The listing builds one solid part. Answer for the finished solid, in the listing's coordinates (mm). A direction names the side the tool comes from. Give positions to 0.01 mm unless a question says otherwise; leave off trailing zeros. Order: outer loops, then holes, each group sorted by start corner. A loop starts at its lowest first (then second) coordinate and runs counter-clockwise, first axis right, second up. Notation, with made-up numbers: (2.25, 43) - (17.25, 43) arc R23 cw to (17.25, 74) - close; hole circle Ø3 at (75, 28). An arc over 180 degrees is marked (long way). Use a Markdown table: item, result. Add a question column.
1) The mould has two halves that part along X. Classify faces 1 (the face through (95.25, 7, 48)), 2 (the face through (8, 13, 74.885)), 3 (the face through (65.55, 4.7, 34.19)), 4 (the face through (0.724, 4.829, 94.486)): released by +X, released by -X, zero draft, split by the parting line, or undercut.
2) Find section A-A, the plane y = 12.75. Determine the outline of the cut face in (x, z) (3 decimals).
3) Flat-ended cylindrical pins translate along their axes: pin 1 (4 mm diameter, centred on x = 89.5, y = 15, fed in from -Z); pin 2 (11 mm diameter, centred on x = 9.525, z = 85.725, fed in from +Y) (3 decimals); pin 3 (3.5 mm diameter, centred on x = 11, z = 45.5, fed in from -Y). Find the tip coordinate at first contact, or state that the pin passes through.
4) Find section B-B, the plane x = 84.5. State how many separate pieces and enclosed holes the cut face has, plus the area to 3 significant figures.
5) Straight lines are drawn through the part: line 1 (Z direction, x = 47.5, y = 16.75) (3 decimals); line 2 (X direction, y = 1.5, z = 43) (3 decimals); line 3 (X direction, y = 9, z = 83). For each, find the intervals that lie inside material, in ascending order.
6) For faces 5 (the face through (46, 6.35, 13)), 6 (the face through (87, 13, 74.885)), 7 (the face through (8, 13, 20.365)), determine the directions among +Z, -Z, +X, -X, +Y, -Y from which every point of the face is accessible in a straight line to the end or side of a thin tool.
from build123d import *

# Parameters (mm, degrees)
SKETCH1_W           = 95.25
SKETCH1_H           = 95.25
SKETCH1_R           = 4.7625
BOSS_EXTRUDE1_DEPTH = 9.525
FILLET1_R           = 2.54
SKETCH3_W           = 54.519743878
SKETCH3_H           = 15.875
SKETCH3_W_2         = 15.875
SKETCH3_H_2         = 54.519743878
BOSS_EXTRUDE3_DEPTH = 7.9375
SKETCH4_R           = 3.3734375
CUT_EXTRUDE1_DEPTH  = 18.4625
SKETCH5_R           = 3.3734375
SKETCH5_W           = 0.508
SKETCH5_H           = 6.745760546
SKETCH5_W_2         = 6.745760546
SKETCH5_H_2         = 0.508
CUT_EXTRUDE2_DEPTH  = 6.35


with BuildPart() as part:
    # Sketch1 → Boss-Extrude1 (new body)
    with BuildSketch(Plane(origin=(0, 0, 0), x_dir=(1, 0, 0), z_dir=(0, 1, 0))):
        with Locations((47.625, -47.625)):
            Rectangle(SKETCH1_W, SKETCH1_H)
        with Locations((9.525, -85.725)):
            Circle(SKETCH1_R, mode=Mode.SUBTRACT)
        Polygon((15.875, -74.884871939), (15.875, -20.365128061), (43.134871939, -47.625), align=None, mode=Mode.SUBTRACT)
        with Locations((85.725, -85.725)):
            Circle(SKETCH1_R, mode=Mode.SUBTRACT)
        Polygon((74.884871939, -79.375), (20.365128061, -79.375), (47.625, -52.115128061), align=None, mode=Mode.SUBTRACT)
        with Locations((9.525, -9.525)):
            Circle(SKETCH1_R, mode=Mode.SUBTRACT)
        Polygon((52.115128061, -47.625), (79.375, -20.365128061), (79.375, -74.884871939), align=None, mode=Mode.SUBTRACT)
        Polygon((47.625, -43.134871939), (20.365128061, -15.875), (74.884871939, -15.875), align=None, mode=Mode.SUBTRACT)
        with Locations((85.725, -9.525)):
            Circle(SKETCH1_R, mode=Mode.SUBTRACT)
    extrude(amount=BOSS_EXTRUDE1_DEPTH)

    # Fillet1
    fillet1_edges = [part.edges().sort_by_distance(p)[0] for p in [
        (95.25, 4.7625, 95.25),
        (0, 4.7625, 95.25),
        (0, 4.7625, 0),
        (95.25, 4.7625, 0),
    ]]
    fillet(fillet1_edges, radius=FILLET1_R)

    # Sketch3 → Boss-Extrude3 (add)
    with BuildSketch(Plane(origin=(0, 9.525, 0), x_dir=(1, 0, 0), z_dir=(0, 1, 0))):
        with Locations((47.625, -7.9375)):
            Rectangle(SKETCH3_W, SKETCH3_H)
        with Locations((87.3125, -47.625)):
            Rectangle(SKETCH3_W_2, SKETCH3_H_2)
        with Locations((47.625, -87.3125)):
            Rectangle(SKETCH3_W, SKETCH3_H)
        with Locations((7.9375, -47.625)):
            Rectangle(SKETCH3_W_2, SKETCH3_H_2)
    extrude(amount=BOSS_EXTRUDE3_DEPTH)

    # Sketch4 → Cut-Extrude1 (cut, through all)
    with BuildSketch(Plane(origin=(0, 17.4625, 0), x_dir=(1, 0, 0), z_dir=(0, 1, 0))):
        with Locations((85.725, -47.625)):
            Circle(SKETCH4_R)
        with Locations((47.625, -85.725)):
            Circle(SKETCH4_R)
        with Locations((9.525, -47.625)):
            Circle(SKETCH4_R)
        with Locations((47.625, -9.525)):
            Circle(SKETCH4_R)
    extrude(amount=-CUT_EXTRUDE1_DEPTH, mode=Mode.SUBTRACT)

    # Sketch5 → Cut-Extrude2 (cut)
    with BuildSketch(Plane.XZ):
        Polygon((85.725, 54.370760545), (79.883, 50.997880273), (79.883, 44.252119727), (85.725, 40.879239455), (91.567, 44.252119727), (91.567, 50.997880273), align=None)
        with Locations((85.725, 47.625)):
            Circle(SKETCH5_R, mode=Mode.SUBTRACT)
        with Locations((79.629, 47.625)):
            Rectangle(SKETCH5_W, SKETCH5_H)
        Polygon((50.997880273, 91.567), (44.252119727, 91.567), (40.879239455, 85.725), (44.252119727, 79.883), (50.997880273, 79.883), (54.370760545, 85.725), align=None)
        with Locations((47.625, 85.725)):
            Circle(SKETCH5_R, mode=Mode.SUBTRACT)
        with Locations((47.625, 79.629)):
            Rectangle(SKETCH5_W_2, SKETCH5_H_2)
        Polygon((15.367, 44.252119727), (15.367, 50.997880273), (9.525, 54.370760545), (3.683, 50.997880273), (3.683, 44.252119727), (9.525, 40.879239455), align=None)
        with Locations((9.525, 47.625)):
            Circle(SKETCH5_R, mode=Mode.SUBTRACT)
        with Locations((15.621, 47.625)):
            Rectangle(SKETCH5_W, SKETCH5_H)
        Polygon((50.997880273, 15.367), (44.252119727, 15.367), (40.879239455, 9.525), (44.252119727, 3.683), (50.997880273, 3.683), (54.370760545, 9.525), align=None)
        with Locations((47.625, 9.525)):
            Circle(SKETCH5_R, mode=Mode.SUBTRACT)
        with Locations((47.625, 15.621)):
            Rectangle(SKETCH5_W_2, SKETCH5_H_2)
    extrude(amount=-CUT_EXTRUDE2_DEPTH, mode=Mode.SUBTRACT)


solid = part.part
The answers:
| question | item | result |
|---|---|---|
| 1 | face 1 | released by +X |
| 1 | face 2 | zero draft |
| 1 | face 3 | undercut |
| 1 | face 4 | released by -X |
| 2 | outline | (0, 20.365) - (15.875, 20.365) - (15.875, 74.885) - (0, 74.885) - close; (20.365, 0) - (74.885, 0) - (74.885, 15.875) - (20.365, 15.875) - close; (20.365, 79.375) - (74.885, 79.375) - (74.885, 95.25) - (20.365, 95.25) - close; (79.375, 20.365) - (95.25, 20.365) - (95.25, 74.885) - (79.375, 74.885) - close; hole circle Ø6.747 at (9.525, 47.625); hole circle Ø6.747 at (47.625, 9.525); hole circle Ø6.747 at (47.625, 85.725); hole circle Ø6.747 at (85.725, 47.625) |
| 3 | pin 1 | z = 20.37 |
| 3 | pin 2 | y = 9.525 |
| 3 | pin 3 | y = 6.35 |
| 4 | separate pieces | 4 |
| 4 | enclosed holes | 0 |
| 4 | area | 1,020 mm2 |
| 5 | line 1 | 0 to 6.154, 12.896 to 15.875, 79.375 to 82.354, 89.096 to 95.25 |
| 5 | line 2 | 0 to 5.852, 13.198 to 15.875, 38.51 to 47.49, 47.76 to 56.74, 79.375 to 82.052, 89.398 to 95.25 |
| 5 | line 3 | 0 to 5.62, 13.43 to 45.64, 49.61 to 81.82, 89.63 to 95.25 |
| 6 | face 5 | -Y |
| 6 | face 6 | +Z, +X, -X, +Y |
| 6 | face 7 | -Z, +X, -X, +Y |
